from build123d import *

# Parameters (mm, degrees)
SKETCH_1_W               = 95
SKETCH_1_H               = 53
EXTRUDE_1_DEPTH          = 2
CUT_EXTRUDE_1_DEPTH      = 55.428852643
CUT_EXTRUDE_1_DEPTH_BACK = 55.428852643


with BuildPart() as part:
    # 草图1 → 凸台-拉伸1 (new, symmetric)
    with BuildSketch(Plane.XY):
        Rectangle(SKETCH_1_W, SKETCH_1_H)
    extrude(amount=EXTRUDE_1_DEPTH, both=True)

    # 草图2 → 切除-拉伸1 (cut, two sides: drawn at the far end of the back side and taken through both)
    with BuildSketch(Plane(origin=(0, 0, 0), x_dir=(1, 0, 0), z_dir=(0, 1, 0)).offset(-CUT_EXTRUDE_1_DEPTH_BACK)):
        Polygon((-131.918074298, -17.94180743), (27.5, -2), (47.5, 0), (27.5, 2), (-131.918074298, 17.94180743), (188.508289392, 17.94180743), (188.508289392, -17.94180743), align=None)
    extrude(amount=CUT_EXTRUDE_1_DEPTH + CUT_EXTRUDE_1_DEPTH_BACK, mode=Mode.SUBTRACT)


solid = part.part
The listing builds one solid part. Answer for the finished solid, in the listing's coordinates (mm). Give positions to 0.01 mm unless a question says otherwise; leave off trailing zeros. Order: outer loops, then holes, each group sorted by start corner. A loop starts at its lowest first (then second) coordinate and runs counter-clockwise, first axis right, second up. Notation, with made-up numbers: (13.5, -39) - (28.5, -39) arc R12 cw to (28.5, -17) - close; hole circle Ø5 at (71, 76). An arc over 180 degrees is marked (long way). One line per item, written item: value. Start each with the question number.
1) A cutting plane is placed at A-A on y = -14. Give the vertices of the cut face in (x, z), then the cut area to 3 significant figures.
2) A cutting plane is placed at B-B on z = 0.7. Give the vertices of the cut face in (x, y), then the cut area to 3 significant figures.
3) Find the intervals of material crossed by L1, parallel to Z at x = 40, y = -20; L2, parallel to Z at x = 30, y = 2.5, in increasing order.
Answer sheet:
1. outline: (-47.5, -2) - (27.5, -2) - (47.5, 0) - (27.5, 2) - (-47.5, 2) - close
1. area: 340 mm2
2. outline: (-47.5, -26.5) - (40.5, -26.5) - (40.5, 26.5) - (-47.5, 26.5) - close
2. area: 4,660 mm2
3. L1: z = -0.75 to 0.75
3. L2: z = -1.75 to 1.75
